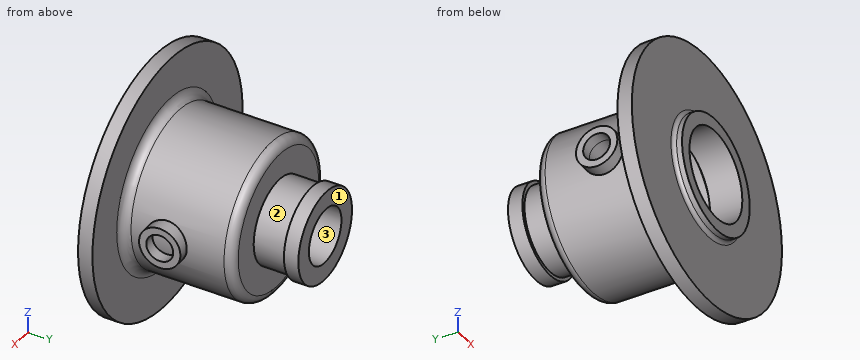
```python
from build123d import *

# Parameters (mm, degrees)
SKETCH2_R           = 11.5
SKETCH2_R_2         = 7.5
BOSS_EXTRUDE1_DEPTH = 10
SKETCH4_R           = 7.5
CUT_EXTRUDE4_DEPTH  = 34
FILLET1_R           = 5
CHAMFER1_SIZE       = 2


# Read off the part's stored shape, not the designer's step: Revolve1
with BuildPart() as part:
    # Revolve1 outline → Revolve1 (revolve)
    with BuildSketch(Plane.XY):
        with BuildLine():
            Line((35, 18), (30, 18))
            ThreePointArc((30, 18), (26.464466094, 16.535533906), (25, 13))
            Line((25, 13), (25, 0))
            Line((25, 0), (32, 0))
            Line((32, 0), (32, 3))
            ThreePointArc((32, 3), (32.585786438, 4.414213562), (34, 5))
            Line((34, 5), (71, 5))
            Line((71, 5), (71, 13))
            Line((71, 13), (48, 13))
            ThreePointArc((48, 13), (44.464466094, 14.464466094), (43, 18))
            Line((43, 18), (43, 74.7))
            Line((43, 74.7), (23.4, 74.7))
            Line((23.4, 74.7), (23.4, 92.7))
            Line((23.4, 92.7), (25.4, 92.7))
            Line((25.4, 92.7), (25.4, 100.7))
            Line((25.4, 100.7), (15.4, 100.7))
            Line((15.4, 100.7), (15.4, 64.7))
            Line((15.4, 64.7), (23.4, 64.7))
            Line((23.4, 64.7), (23.4, 66.7))
            Line((23.4, 66.7), (35, 66.7))
            Line((35, 66.7), (35, 18))
        make_face()
    revolve(axis=Axis((0, 0, 0), (0, 1, 0)))



with BuildPart() as body_2:
    # Revolve1 2 outline → Revolve1 2 (revolve)
    with BuildSketch(Plane.XY):
        with BuildLine():
            Line((15.4, 100.7), (15.4, 64.7))
            Line((15.4, 64.7), (23.4, 64.7))
            Line((23.4, 64.7), (23.4, 66.7))
            Line((23.4, 66.7), (35, 66.7))
            Line((35, 66.7), (35, 23))
            ThreePointArc((35, 23), (33.535533906, 19.464466094), (30, 18))
            Line((30, 18), (25, 18))
            Line((25, 18), (25, 0))
            Line((25, 0), (32, 0))
            Line((32, 0), (32, 3))
            ThreePointArc((32, 3), (32.585786438, 4.414213562), (34, 5))
            Line((34, 5), (71, 5))
            Line((71, 5), (71, 13))
            Line((71, 13), (48, 13))
            ThreePointArc((48, 13), (44.464466094, 14.464466094), (43, 18))
            Line((43, 18), (43, 74.7))
            Line((43, 74.7), (23.4, 74.7))
            Line((23.4, 74.7), (23.4, 92.7))
            Line((23.4, 92.7), (25.4, 92.7))
            Line((25.4, 92.7), (25.4, 100.7))
            Line((25.4, 100.7), (15.4, 100.7))
        make_face()
    revolve(axis=Axis((0, 0, 0), (0, 1, 0)))


with BuildPart() as part_1:
    add(part.part)

    add(body_2.part)  # Boss-Extrude1 merges body 2
    # Sketch2 → Boss-Extrude1 (add)
    with BuildSketch(Plane(origin=(-49, 0, 0), x_dir=(0, 0, -1), z_dir=(1, 0, 0))):
        with Locations(Location((0, 37.5, 0), (0, 0, 180))):
            Circle(SKETCH2_R)
        with Locations(Location((0, 37.5, 0), (0, 0, 180))):
            Circle(SKETCH2_R_2, mode=Mode.SUBTRACT)
    boss_extrude1 = extrude(amount=BOSS_EXTRUDE1_DEPTH)

    # Sketch4 → Cut-Extrude4 (cut)
    with BuildSketch(Plane(origin=(-49, 0, 0), x_dir=(0, 0, -1), z_dir=(1, 0, 0))):
        with Locations(Location((0, 37.5, 0), (0, 0, 180))):
            Circle(SKETCH4_R)
    extrude(amount=CUT_EXTRUDE4_DEPTH, mode=Mode.SUBTRACT)

    # Mirror1: Boss-Extrude1 across plane
    add(boss_extrude1.mirror(Plane(origin=(0, 0, 0), x_dir=(0, 0, 1), z_dir=(1, 0, 0))))

    # Fillet1
    fillet1_edges = [part_1.edges().sort_by_distance(p)[0] for p in [
        (-43, 74.7, 0),
    ]]
    fillet(fillet1_edges, radius=FILLET1_R)

    # Chamfer1
    chamfer1_edges = [part_1.edges().sort_by_distance(p)[0] for p in [
        (-15.4, 64.7, 0),
    ]]
    chamfer(chamfer1_edges, length=CHAMFER1_SIZE)


solid = part_1.part
```
Input: part model. Units: mm. Frame: model coordinates. Face numbers are marked on the shaded views. Give positions to 0.01 mm unless a question says otherwise; leave off trailing zeros. Order: outer loops, then holes, each group sorted by start corner. A loop starts at its lowest first (then second) coordinate and runs counter-clockwise, first axis right, second up. Notation, with made-up numbers: (-16, 30.25) - (18, 30.25) arc R13 cw to (18, 38.25) - close; hole circle Ø5 at (74.25, 31). An arc over 180 degrees is marked (long way). Use a Markdown table: item, result.
(1) Draft query along Y for the marked faces 1, 2 and 3. Return one class per face: released by +Y, released by -Y, zero draft, split by the parting line, or undercut.
Computed values:
| item | result |
|---|---|
| face 1 | released by +Y |
| face 2 | undercut |
| face 3 | zero draft |
(2) Section query B-B (y = 86). Output: boundary loops of the cut face in (x, z), then the cut area to 3 significant figures.
Computed values:
| item | result |
|---|---|
| outline | circle Ø46.8 at (0, 0); hole circle Ø30.8 at (0, 0) |
| area | 975 mm2 |
(3) Section query D-D (x = 53). Output: boundary loops of the cut face in (y, z), then the cut area to 3 significant figures.
Computed values:
| item | result |
|---|---|
| outline | (5, -47.24) - (13, -47.24) - (13, 47.24) - (5, 47.24) - close |
| area | 756 mm2 |
(4) Section query C-C (z = 0). State how many separate pieces and enclosed holes the cut face has, then the cut area to 3 significant figures.
Computed values:
| item | result |
|---|---|
| separate pieces | 3 |
| enclosed holes | 0 |
| area | 2,670 mm2 |
(5) Section query A-A (y = 37.5). Output: boundary loops of the cut face in (x, z).
Computed values:
| item | result |
|---|---|
| outline | (-49, -11.5) - (-41.43, -11.5) arc R43 ccw to (41.43, -11.5) - (49, -11.5) - (49, -7.5) - (42.34, -7.5) arc R43 ccw to (42.34, 7.5) - (49, 7.5) - (49, 11.5) - (41.43, 11.5) arc R43 ccw to (-41.43, 11.5) - (-49, 11.5) - (-49, 7.5) - (-34.19, 7.5) arc R35 cw (long way) to (-34.19, -7.5) - (-49, -7.5) - close |
(6) Pin query (flat end, axial travel): pin 1 (3 mm diameter, centred on x = -30, z = 28.5, fed in from +Y); pin 2 (1.5 mm diameter, centred on y = 78.5, z = 11.5, fed in from +X); pin 3 (7 mm diameter, centred on y = 36, z = 2.5, fed in from -X). Return the tip coordinate at first contact, or that it passes through.
Computed values:
| item | result |
|---|---|
| pin 1 | stops at y = 74.33 |
| pin 2 | stops at x = 20.78 |
| pin 3 | stops at x = 34.48 |
(7) Line query: line 1 (Y direction, x = 47.5, z = 0); line 2 (Z direction, x = 0, y = 51). Output: solid intervals per line, ascending. Write a range as from..to.
Computed values:
| item | result |
|---|---|
| line 1 | y = 5..13.03, 26..30, 45..49 |
| line 2 | z = -43..-35, 35..43 |
